Could you check a few things on this model? Use its own coordinates, in mm. Face numbers are marked on the shaded views. Round coordinates to 2 decimals unless told otherwise and drop trailing zeros. Write each loop counter-clockwise with the first axis right and the second up, starting at its lowest first coordinate (ties: lowest second). Pieces come first, ordered by that corner, then holes.
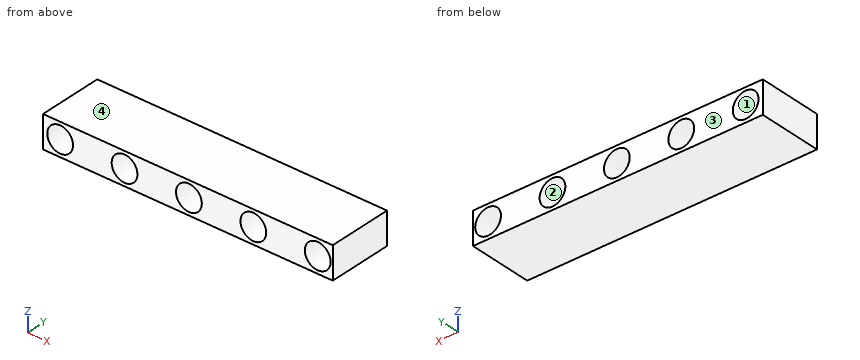
```python
from build123d import *

# Parameters (mm, degrees)
SKETCH_1_W          = 50
SKETCH_1_H          = 5
SKETCH_1_R          = 2
EXTRUDE_1_DEPTH     = 10
SKETCH_2_W          = 4.996058956
SKETCH_2_H          = 5
CUT_EXTRUDE_1_DEPTH = 10


with BuildPart() as part:
    # 草图1 → 凸台-拉伸1 (new body)
    with BuildSketch(Plane(origin=(0, 0, 0), x_dir=(1, 0, 0), z_dir=(0, 1, 0))):
        with Locations((-15, 0)):
            Rectangle(SKETCH_1_W, SKETCH_1_H)
        with Locations(Location((-37.33819922, 0, 0), (0, 0, 270))):
            Circle(SKETCH_1_R, mode=Mode.SUBTRACT)
        with Locations(Location((-27.33819922, 0, 0), (0, 0, 270))):
            Circle(SKETCH_1_R, mode=Mode.SUBTRACT)
        with Locations(Location((-17.33819922, 0, 0), (0, 0, 270))):
            Circle(SKETCH_1_R, mode=Mode.SUBTRACT)
        with Locations(Location((-7.33819922, 0, 0), (0, 0, 270))):
            Circle(SKETCH_1_R, mode=Mode.SUBTRACT)
        with Locations(Location((2.66180078, 0, 0), (0, 0, 270))):
            Circle(SKETCH_1_R, mode=Mode.SUBTRACT)
    extrude(amount=EXTRUDE_1_DEPTH)

    # 草图2 → 切除-拉伸1 (cut)
    with BuildSketch(Plane(origin=(0, 10, 0), x_dir=(1, 0, 0), z_dir=(0, 1, 0))):
        with Locations((7.501970522, 0)):
            Rectangle(SKETCH_2_W, SKETCH_2_H)
    extrude(amount=-CUT_EXTRUDE_1_DEPTH, mode=Mode.SUBTRACT)


solid = part.part
```
Q1. If I drill on L1, parallel to X at y = 4.75, z = 0; L2, parallel to X at y = 5.75, z = -1.2; L3, parallel to Z at x = 1.5, y = 7.25, over which ranges is the centre line in solid material (lowest first)?
Q2. We'd pull the mould along Z, two halves only. Please class the marked faces 1, 2, 3 and 4: pulls with the +Z half, pulls with the -Z half, needs draft (parallel to the pull), parting line crosses it, or undercut.
Q3. Imagine slicing it at C-C, the plane y = 5. Write out the boundary of the cut face in (x, z), then the cut area to 3 significant figures.
Q4. Imagine slicing it at A-A, the plane z = 0. Write out the boundary of the cut face in (x, y).
Q5. Imagine slicing it at B-B, the plane x = 1.5. Write out the boundary of the cut face in (y, z).
Results found:
1. L1: x = -40 to -39.34, -35.34 to -29.34, -25.34 to -19.34, -15.34 to -9.34, -5.34 to 0.66, 4.66 to 5
1. L2: x = -40 to -38.94, -35.74 to -28.94, -25.74 to -18.94, -15.74 to -8.94, -5.74 to 1.06, 4.26 to 5
1. L3: z = -2.5 to -1.63, 1.63 to 2.5
2. face 1: undercut
2. face 2: undercut
2. face 3: needs draft
2. face 4: pulls with the +Z half
3. outline: (-40, -2.5) - (5, -2.5) - (5, 2.5) - (-40, 2.5) - close; hole circle Ø4 at (-37.34, 0); hole circle Ø4 at (-27.34, 0); hole circle Ø4 at (-17.34, 0); hole circle Ø4 at (-7.34, 0); hole circle Ø4 at (2.66, 0)
3. area: 162 mm2
4. outline: (-40, 0) - (-39.34, 0) - (-39.34, 10) - (-40, 10) - close; (-35.34, 0) - (-29.34, 0) - (-29.34, 10) - (-35.34, 10) - close; (-25.34, 0) - (-19.34, 0) - (-19.34, 10) - (-25.34, 10) - close; (-15.34, 0) - (-9.34, 0) - (-9.34, 10) - (-15.34, 10) - close; (-5.34, 0) - (0.66, 0) - (0.66, 10) - (-5.34, 10) - close; (4.66, 0) - (5, 0) - (5, 10) - (4.66, 10) - close
5. outline: (0, -2.5) - (10, -2.5) - (10, -1.63) - (0, -1.63) - close; (0, 1.63) - (10, 1.63) - (10, 2.5) - (0, 2.5) - close
